CAD build for the part. Positions are in the model's coordinates, mm. Face numbers are marked on the shaded views. A direction names the side the tool comes from. Give positions to 0.01 mm unless a question says otherwise; leave off trailing zeros. Loops run counter-clockwise (first coordinate to the right, second up) from the corner with the lowest first, then second, coordinate; pieces in that order, holes last. Notation, with made-up numbers: M 46.25,45.25 L 63.25,45.25 A13 ccw 63.25,55.25 Z; hole C 9,30 d2. An arc over 180 degrees is marked long. Answer as CSV lines item,"result".
from build123d import *

# Parameters (mm, degrees)
EXTRUDE_1_DEPTH     = 1.3
FILLET_1_R          = 3
SKETCH_2_W          = 1.3
SKETCH_2_H          = 6
EXTRUDE_2_DEPTH     = 14
FILLET_2_R          = 3
SKETCH_3_W          = 1.3
SKETCH_3_H          = 7.65
EXTRUDE_3_DEPTH     = 7
SKETCH_4_W          = 1.3
SKETCH_4_H          = 4.35
EXTRUDE_4_DEPTH     = 7
FILLET_3_R          = 3
FILLET_4_R          = 5
SKETCH_6_W          = 1.3
SKETCH_6_H          = 6
EXTRUDE_5_DEPTH     = 13
SKETCH_7_W          = 1.3
SKETCH_7_H          = 13
EXTRUDE_6_DEPTH     = 8
FILLET_5_R          = 3
FILLET_6_R          = 5
SKETCH_8_R          = 1.6
SKETCH_8_R_2        = 2
CUT_EXTRUDE_1_DEPTH = 8
SKETCH_9_R          = 7.5
EXTRUDE_7_DEPTH     = 10
SKETCH_10_R         = 1.5
EXTRUDE_10_DEPTH    = 139


with BuildPart() as part:
    # 草图1 → 凸台-拉伸1 (new body)
    with BuildSketch(Plane.XY):
        Polygon((-71, 0), (0, 0), (71, 0), (71, 6), (67, 6), (67, 18), (-67, 18), (-67, 6), (-71, 6), align=None)
    extrude(amount=-EXTRUDE_1_DEPTH)

    # 圆角1
    fillet_1_edges = [part.edges().sort_by_distance(p)[0] for p in [
        (-67, 18, -0.65),
        (67, 18, -0.65),
    ]]
    fillet(fillet_1_edges, radius=FILLET_1_R)

    # 草图2 → 凸台-拉伸2 (add)
    with BuildSketch(Plane.XY):
        with Locations((-70.35, 3)):
            Rectangle(SKETCH_2_W, SKETCH_2_H)
    extrude(amount=EXTRUDE_2_DEPTH)

    # 圆角2
    fillet_2_edges = [part.edges().sort_by_distance(p)[0] for p in [
        (-70.35, 6, 14),
    ]]
    fillet(fillet_2_edges, radius=FILLET_2_R)

    # 草图3 → 凸台-拉伸3 (add)
    with BuildSketch(Plane.XZ):
        with Locations((-70.35, 10.175)):
            Rectangle(SKETCH_3_W, SKETCH_3_H)
    extrude(amount=EXTRUDE_3_DEPTH)

    # 草图4 → 凸台-拉伸4 (add)
    with BuildSketch(Plane.XZ):
        with Locations((-70.35, 4.175)):
            Rectangle(SKETCH_4_W, SKETCH_4_H)
    extrude(amount=EXTRUDE_4_DEPTH)

    # 圆角3
    fillet_3_edges = [part.edges().sort_by_distance(p)[0] for p in [
        (-70.35, -7, 14),
    ]]
    fillet(fillet_3_edges, radius=FILLET_3_R)

    # 圆角4
    fillet_4_edges = [part.edges().sort_by_distance(p)[0] for p in [
        (-70.35, -7, 2),
    ]]
    fillet(fillet_4_edges, radius=FILLET_4_R)

    # 草图6 → 凸台-拉伸5 (add)
    with BuildSketch(Plane.XY):
        with Locations((70.35, 3)):
            Rectangle(SKETCH_6_W, SKETCH_6_H)
    extrude(amount=EXTRUDE_5_DEPTH)

    # 草图7 → 凸台-拉伸6 (add)
    with BuildSketch(Plane.XZ):
        with Locations((70.35, 6.5)):
            Rectangle(SKETCH_7_W, SKETCH_7_H)
    extrude(amount=EXTRUDE_6_DEPTH)

    # 圆角5
    fillet_5_edges = [part.edges().sort_by_distance(p)[0] for p in [
        (70.35, 6, 13),
        (70.35, -8, 13),
    ]]
    fillet(fillet_5_edges, radius=FILLET_5_R)

    # 圆角6
    fillet_6_edges = [part.edges().sort_by_distance(p)[0] for p in [
        (70.35, -8, 0),
    ]]
    fillet(fillet_6_edges, radius=FILLET_6_R)

    # 草图8 → 切除-拉伸1 (cut)
    with BuildSketch(Plane.XY):
        with Locations((-56, 12)):
            Circle(SKETCH_8_R)
        with Locations((-46, 12)):
            Circle(SKETCH_8_R_2)
        with Locations((-9, 12)):
            Circle(SKETCH_8_R)
        with Locations((59, 12)):
            Circle(SKETCH_8_R)
        with BuildLine():
            Line((42.5, 14.5), (47.5, 14.5))
            ThreePointArc((47.5, 14.5), (50, 12), (47.5, 9.5))
            Line((47.5, 9.5), (42.5, 9.5))
            ThreePointArc((42.5, 9.5), (40, 12), (42.5, 14.5))
        make_face()
    extrude(amount=-CUT_EXTRUDE_1_DEPTH, mode=Mode.SUBTRACT)

    # 草图9 → 凸台-拉伸7 (add)
    with BuildSketch(Plane(origin=(71, 0, 0), x_dir=(0, 0, -1), z_dir=(1, 0, 0))):
        with Locations((-7.5, -1)):
            Circle(SKETCH_9_R)
    extrude(amount=EXTRUDE_7_DEPTH)

    # 草图10 → 凸台-拉伸10 (add)
    with BuildSketch(Plane.ZY.offset(-69.7)):
        with Locations((9.5, 2.5)):
            Circle(SKETCH_10_R)
        with Locations((9.5, -2.5)):
            Circle(SKETCH_10_R)
        with Locations((3, 0)):
            Circle(SKETCH_10_R)
    extrude(amount=EXTRUDE_10_DEPTH)


solid = part.part
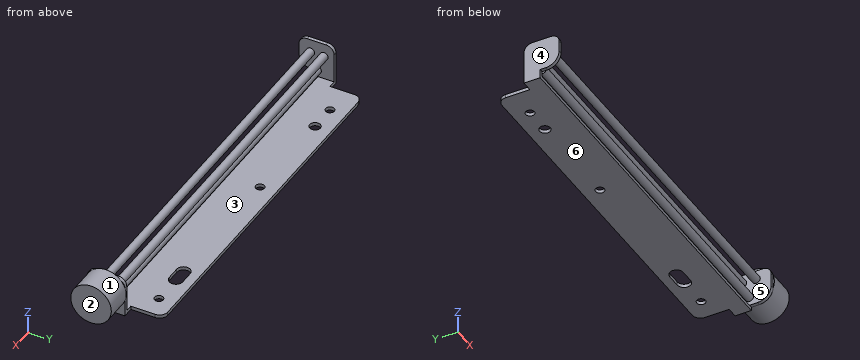
1) Band-saw the part on D-D on x = -46. Give the cut face in (y, z), and give its area (3 significant figures).
Answer below:
outline,"C -2.5,9.5 d3; C 0,3 d3; M 0,-1.3 L 10,-1.3 L 10,0 L 0,0 Z; C 2.5,9.5 d3; M 14,-1.3 L 18,-1.3 L 18,0 L 14,0 Z"
area,"39.4 mm^2"
2) Band-saw the part on B-B on x = 18.5. Give the cut face in (y, z), and give its area (3 significant figures).
Answer below:
outline,"C -2.5,9.5 d3; C 0,3 d3; M 0,-1.3 L 18,-1.3 L 18,0 L 0,0 Z; C 2.5,9.5 d3"
area,"44.6 mm^2"
3) Which spindle directions (+Z, -Z, +X, -X, +Y, -Y) get a long thin tool onto all of the face, cutting with end or side? Do the marked faces 1, 2 and 3. Say none if no direction does.
Answer below:
face 1,"+X"
face 2,"+Z, -Z, +X, +Y, -Y"
face 3,"+Y, -Y"
4) Mould opens along X. For the marked faces 4, 5 and 6 say: +X half, -X half, draft (parallel to the pull), parting line (faces both ways), or undercut.
Answer below:
face 4,"-X half"
face 5,"undercut"
face 6,"draft"
5) Flat gauge pins, fed straight in: pin 1 (1.5 mm diameter, centred on y = 13, z = 1, fed in from +X) (3 decimals); pin 2 (1.4 mm diameter, centred on x = 70.5, y = -2, fed in from -Z); pin 3 (3 mm diameter, centred on x = -16.5, y = -2, fed in from +Z); pin 4 (1.4 mm diameter, centred on y = 8.5, z = -0.5, fed in from +X). Where does each tip first touch, or does it go through?
Answer below:
pin 1,"passes through"
pin 2,"stops at z = 0"
pin 3,"stops at z = 11"
pin 4,"stops at x = 67"
6) Band-saw the part on C-C on x = 59. Give the cut face in (y, z), and give its area (3 significant figures).
Answer below:
outline,"C -2.5,9.5 d3; C 0,3 d3; M 0,-1.3 L 10.4,-1.3 L 10.4,0 L 0,0 Z; C 2.5,9.5 d3; M 13.6,-1.3 L 18,-1.3 L 18,0 L 13.6,0 Z"
area,"40.4 mm^2"
7) Band-saw the part on A-A on y = 12. Give the cut face in (x, z).
Answer below:
outline,"M -67,-1.3 L -57.6,-1.3 L -57.6,0 L -67,0 Z; M -54.4,-1.3 L -48,-1.3 L -48,0 L -54.4,0 Z; M -44,-1.3 L -10.6,-1.3 L -10.6,0 L -44,0 Z; M -7.4,-1.3 L 40,-1.3 L 40,0 L -7.4,0 Z; M 50,-1.3 L 57.4,-1.3 L 57.4,0 L 50,0 Z; M 60.6,-1.3 L 67,-1.3 L 67,0 L 60.6,0 Z"
8) Drill centre lines: line 1 (X direction, y = 3.75, z = 10.5); line 2 (Y direction, x = -9, z = -0.25); line 3 (Y direction, x = -46, z = -0.4). Where is each one in solid material? Low to high. Write a range as from..to.
Answer below:
line 1,"x = -71..-69.7, 69.7..81"
line 2,"y = 0..10.4, 13.6..18"
line 3,"y = 0..10, 14..18"
